Here's the drawing with two shaded views (mm, measured from the low corner). I have some questions. A direction names the side the tool comes from. Give positions to 0.01 mm unless a question says otherwise; leave off trailing zeros. Write each loop counter-clockwise with the first axis right and the second up, starting at its lowest first coordinate (ties: lowest second). Pieces come first, ordered by that corner, then holes.
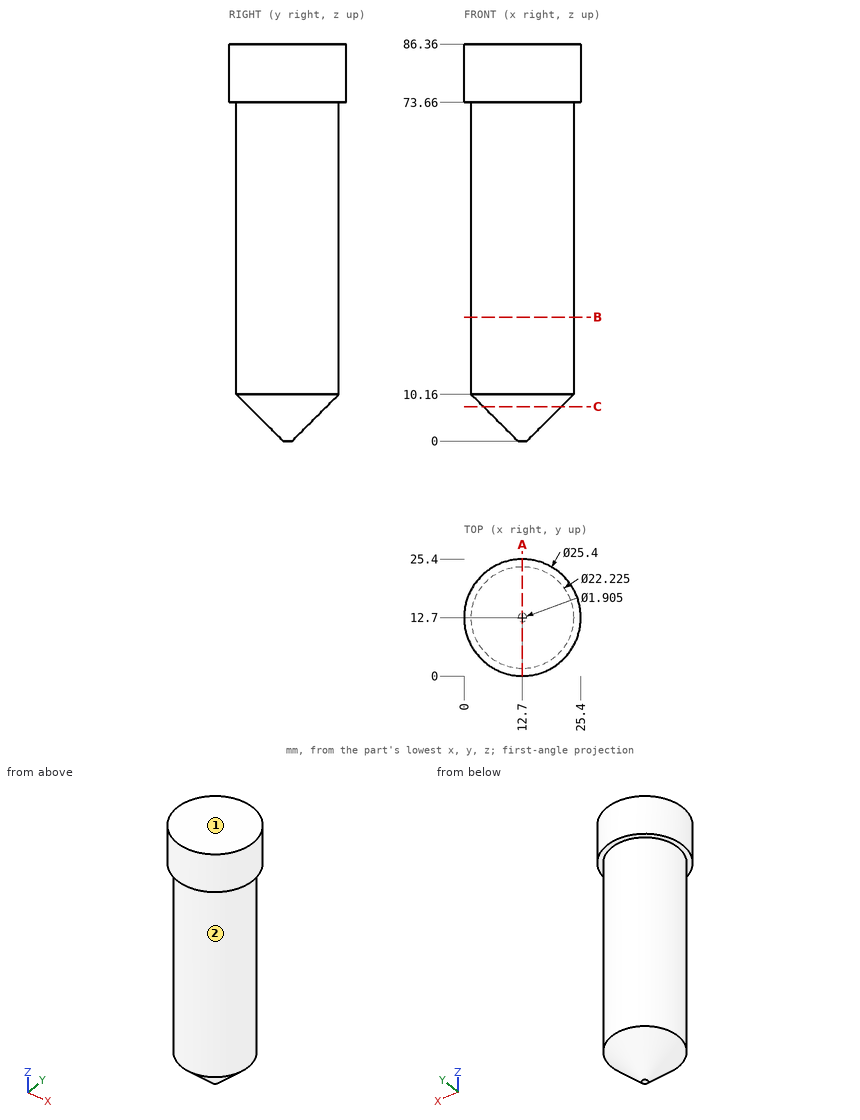
1) For the marked faces 1 and 2, which set-ups out of +Z, -Z, +X, -X, +Y, -Y let a thin tool reach every point of the face, with its end or its side?
Values follow:
face 1: +Z, +X, -X, +Y, -Y
face 2: -Z
2) Suppose I cut it at A-A on x = 12.7. Write out the boundary of the cut face in (y, z), plus the area to 3 significant figures.
Values follow:
outline: (0, 73.66) - (1.59, 73.66) - (1.59, 10.16) - (11.75, 0) - (13.65, 0) - (23.81, 10.16) - (23.81, 73.66) - (25.4, 73.66) - (25.4, 86.36) - (0, 86.36) - close
area: 1,860 mm2
3) Please list where these lines run through material, in increasing order: L1, parallel to Z at x = 24.5, y = 16.5; L2, parallel to X at y = 13.25, z = 11.5; L3, parallel to Y at x = 12.75, z = 25.5.
Values follow:
L1: z = 73.66 to 86.36
L2: x = 1.6 to 23.8
L3: y = 1.59 to 23.81
4) Suppose I cut it at B-B on z = 27. Write out the boundary of the cut face in (x, y) (1 decimal).
Values follow:
outline: circle Ø22.2 at (12.7, 12.7)
5) Suppose I cut it at C-C on z = 7.5. Write out the boundary of the cut face in (x, y) (1 decimal).
Values follow:
outline: circle Ø16.9 at (12.7, 12.7)
6) For pin 1 Ø3 at (x, y) = (22, 10) entering from -Z; pin 2 Ø2 at (y, z) = (23, 58.5) entering from -X; pin 3 Ø4 at (x, z) = (3.5, 17) entering from -Y, each with a flat end and sliding along its axis, tell me the tip position at first contact or that it passes through.
Values follow:
pin 1: stops at z = 7.23
pin 2: stops at x = 6.62
pin 3: stops at y = 4.24
